from build123d import *

# Parameters (mm, degrees)
SCHIZZO1_W                   = 44
SCHIZZO1_H                   = 60
ESTRUSIONE_ESTRUSIONE1_DEPTH = 26
SCHIZZO2_W                   = 21
SCHIZZO2_H                   = 3.8
TAGLIO_ESTRUSIONE1_DEPTH     = 45
RIPETIZIONE_A_L1_COUNT       = 8
RIPETIZIONE_A_L1_PITCH       = 4.82
SCHIZZO3_W                   = 21.5
SCHIZZO3_H                   = 10.23
TAGLIO_ESTRUSIONE2_DEPTH     = 45
TAGLIO_ESTRUSIONE4_DEPTH     = 5.5


with BuildPart() as part:
    # Schizzo1 → Estrusione-Estrusione1 (new body)
    with BuildSketch(Plane.XY):
        Rectangle(SCHIZZO1_W, SCHIZZO1_H)
    extrude(amount=ESTRUSIONE_ESTRUSIONE1_DEPTH)

    # Schizzo2 → Taglio-Estrusione1 (cut, through all)
    with BuildSketch(Plane.ZY.offset(22)):
        with Locations((10.5, -16.85)):
            Rectangle(SCHIZZO2_W, SCHIZZO2_H)
    taglio_estrusione1 = extrude(amount=-TAGLIO_ESTRUSIONE1_DEPTH, mode=Mode.SUBTRACT)

    # Ripetizione a L1: Taglio-Estrusione1 ×8
    with Locations(*[(0, i * RIPETIZIONE_A_L1_PITCH, 0) for i in range(1, RIPETIZIONE_A_L1_COUNT)]):
        add(taglio_estrusione1, mode=Mode.SUBTRACT)

    # Schizzo3 → Taglio-Estrusione2 (cut, through all)
    with BuildSketch(Plane(origin=(22, 0, 0), x_dir=(0, 0, -1), z_dir=(1, 0, 0))):
        with Locations((-10.75, -24.885)):
            Rectangle(SCHIZZO3_W, SCHIZZO3_H)
        with Locations((-10.75, 24.885)):
            Rectangle(SCHIZZO3_W, SCHIZZO3_H)
    extrude(amount=-TAGLIO_ESTRUSIONE2_DEPTH, mode=Mode.SUBTRACT)

    # Schizzo5 → Taglio-Estrusione4 (cut, through all)
    with BuildSketch(Plane(origin=(0, 0, 21.5), x_dir=(-1, 0, 0), z_dir=(0, 0, -1))):
        with BuildLine():
            Line((3.35, 34.5), (3.35, 25.5))
            ThreePointArc((3.35, 25.5), (0, 22.15), (-3.35, 25.5))
            Line((-3.35, 25.5), (-3.35, 34.5))
            ThreePointArc((-3.35, 34.5), (0, 37.85), (3.35, 34.5))
        make_face()
        with BuildLine():
            Line((-3.35, -33.313801036), (-3.35, -26.686198964))
            ThreePointArc((-3.35, -26.686198964), (0, -23.336198964), (3.35, -26.686198964))
            Line((3.35, -26.686198964), (3.35, -33.313801036))
            ThreePointArc((3.35, -33.313801036), (0, -36.663801036), (-3.35, -33.313801036))
        make_face()
    extrude(amount=-TAGLIO_ESTRUSIONE4_DEPTH, mode=Mode.SUBTRACT)


solid = part.part
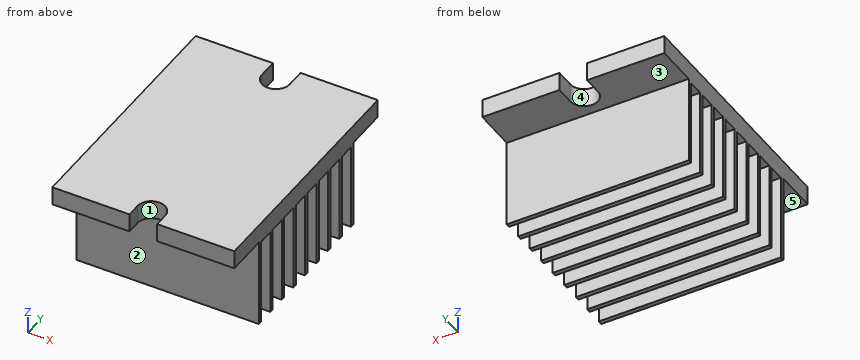
Check sheet for the modelled part. Datum: model origin and axes. Units: mm. Face numbers are marked on the shaded views. A direction names the side the tool comes from. Round coordinates to 2 decimals unless told otherwise and drop trailing zeros. Order: outer loops, then holes, each group sorted by start corner. A loop starts at its lowest first (then second) coordinate and runs counter-clockwise, first axis right, second up.
(1) Access from +Z, -Z, +X, -X, +Y, -Y to the whole of each face (thin tool, end or side, straight path). Record for the marked faces 3, 4 and 5.
(2) Go/stop test with flat-tipped pins: P1, Ø8, axis at x = 0, z = 8, coming from the +Y side; P2, Ø1.1, axis at x = -8, y = -1.5, coming from the -Z side; P3, Ø3, axis at x = 13, z = 9.5, coming from the -Y side. Record where each tip stops, or that it passes through.
(3) Scan lines: probe 1 along Z at (x, y) = (-14, 20); probe 2 along Z at (x, y) = (18, -4). Record each from-to range of solid material in increasing order.
(4) Cross-section at A-A, the plane y = 24. Enter the section's corners in (x, z).
(5) Draft check along X on the marked faces 1 and 2. Enter one of: pulls with the +X half, pulls with the -X half, needs draft (parallel to the pull), parting line crosses it, or undercut.
(6) Cross-section at B-B, the plane z = 5.75. State how many separate pieces and enclosed holes the cut face has, and give its area (3 significant figures).
Check sheet entries:
1. face 3: -Z, +X, -X, +Y
1. face 4: +Z, -Z, +Y
1. face 5: -Z, +X, -X, -Y
2. P1: stops at y = 19.77
2. P2: stops at z = 21
2. P3: stops at y = -19.77
3. probe 1: z = 21.5 to 26
3. probe 2: z = 21 to 26
4. outline: (-22, 21.5) - (-3, 21.5) - (-3, 26) - (-22, 26) - close; (3, 21.5) - (22, 21.5) - (22, 26) - (3, 26) - close
5. face 1: undercut
5. face 2: needs draft
6. separate pieces: 9
6. enclosed holes: 0
6. area: 402 mm2
